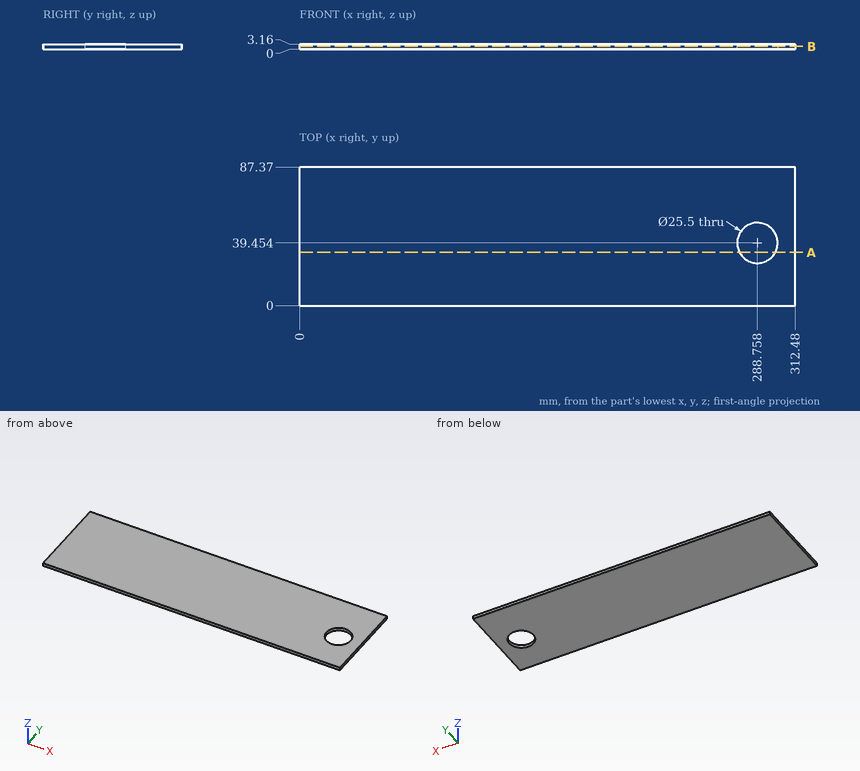
Part print with two shaded views. Sizes in mm from the minimum x, y, z corner. Round coordinates to 2 decimals unless told otherwise and drop trailing zeros. Order: outer loops, then holes, each group sorted by start corner. A loop starts at its lowest first (then second) coordinate and runs counter-clockwise, first axis right, second up. Notation, with made-up numbers: (-7, 46) -> (21, 46) arc R24 cw to (21, 77) -> close; hole circle Ø5 at (-5, -8). An arc over 180 degrees is marked (long way). Write each question's results on one line, items separated by ' | '.
1. Cut at A-A (y = 33.5). Give the cut face in (x, z).
Findings below:
outline: (0, 0) -> (277.48, 0) -> (277.48, 3.16) -> (0, 3.16) -> close; (300.03, 0) -> (312.48, 0) -> (312.48, 3.16) -> (300.03, 3.16) -> close
2. Wall check: line 1 along X through (y, z) = (29.5, 1.95) (1 decimal); line 2 along Y through (x, z) = (277.5, 0.2) (1 decimal); line 3 along X through (y, z) = (34, 2.75) (1 decimal). Give the ranges that are in metal, low to high. Write a range as [from, to].
Findings below:
line 1: x = [0, 280.8], [296.7, 312.5] | line 2: y = [0, 33.5], [45.4, 87.4] | line 3: x = [0, 277.2], [300.3, 312.5]
3. Cut at B-B (z = 1.6). Give the cut face in (x, y), plus the area to 3 significant figures.
Findings below:
outline: (0, 0) -> (312.48, 0) -> (312.48, 87.37) -> (0, 87.37) -> close; hole circle Ø25.5 at (288.76, 39.45) | area: 26,800 mm²
